```python
from build123d import *

# Parameters (mm, degrees)
F0_W     = 25.516171
F0_H     = 19.186575
F1_DEPTH = 50.8


with BuildPart() as f1:
    # F0 (on Front) → F1 (new body)
    with BuildSketch(Plane.XZ):
        with BuildLine():
            ThreePointArc((-72.431024, 58.625113), (-75.125101, 57.50919), (-76.241024, 54.815113))
            Line((-76.241024, 54.815113), (-76.241024, 3.81))
            ThreePointArc((-76.241024, 3.81), (-75.125101, 1.115923), (-72.431024, 0))
            Line((-72.431024, 0), (-65.04178, 0))
            ThreePointArc((-65.04178, 0), (-53.842533, 13.818248), (-42.643286, 0))
            Line((-42.643286, 0), (-8.830175, 0))
            ThreePointArc((-8.830175, 0), (2.476757, 13.272119), (13.783689, 0))
            Line((13.783689, 0), (49.104389, 0))
            Line((49.104389, 0), (49.104389, 27.893852))
            ThreePointArc((49.104389, 27.893852), (47.988466, 30.587929), (45.294389, 31.703852))
            Line((45.294389, 31.703852), (22.183126, 31.703852))
            Line((22.183126, 31.703852), (1.142996, 57.237982))
            ThreePointArc((1.142996, 57.237982), (-0.171807, 58.260924), (-1.797379, 58.625113))
            Line((-1.797379, 58.625113), (-72.431024, 58.625113))
        make_face()
        with Locations((-51.349548, 42.823649)):
            Rectangle(F0_W, F0_H, mode=Mode.SUBTRACT)
        Polygon((-18.218089, 33.230361), (-18.218089, 52.416936), (0, 52.416936), (14.814471, 33.230361), align=None, mode=Mode.SUBTRACT)
    extrude(amount=F1_DEPTH)


solid = f1.part
```
Input: part model. Units: mm. Frame: model coordinates. A direction names the side the tool comes from. Give positions to 0.01 mm unless a question says otherwise; leave off trailing zeros. Order: outer loops, then holes, each group sorted by start corner. A loop starts at its lowest first (then second) coordinate and runs counter-clockwise, first axis right, second up. Notation, with made-up numbers: M -5,11.5 L 28,11.5 A31 cw 28,37.5 Z; hole C 65.5,87.5 d3. An arc over 180 degrees is marked long. Return JSON: item names as keys, results as strings.
1) Mould query, pull axis Z, two halves, no side actions, for faces 1 (the face through (-52, -25, 33.23)), 2 (the face through (34, -25, 31.704)), 3 (the face through (-26, -25, 0)). Classes: released by +Z, released by -Z, zero draft, split by the parting line, or undercut.
Taken from the geometry:
{"face 1": "undercut", "face 2": "released by +Z", "face 3": "released by -Z"}
2) Section query B-B on y = -6. Output: boundary loops of the cut face in (x, z).
Taken from the geometry:
{"outline": "M -76.24,3.81 A3.81 ccw -72.43,0 L -65.04,0 A11.45 cw long -42.64,0 L -8.83,0 A11.45 cw long 13.78,0 L 49.1,0 L 49.1,27.89 A3.81 ccw 45.29,31.7 L 22.18,31.7 L 1.14,57.24 A3.81 ccw -1.8,58.63 L -72.43,58.63 A3.81 ccw -76.24,54.82 Z; hole M -64.11,33.23 L -38.59,33.23 L -38.59,52.42 L -64.11,52.42 Z; hole M -18.22,33.23 L 14.81,33.23 L 0,52.42 L -18.22,52.42 Z"}
3) Section query A-A on z = 35. Output: boundary loops of the cut face in (x, y).
Taken from the geometry:
{"outline": "M -76.24,-50.8 L -64.11,-50.8 L -64.11,0 L -76.24,0 Z; M -38.59,-50.8 L -18.22,-50.8 L -18.22,0 L -38.59,0 Z; M 13.45,-50.8 L 19.47,-50.8 L 19.47,0 L 13.45,0 Z"}
4) Contact query for flat-ended pins moving along their axis: pin 1 (13 mm diameter, centred on x = -50.5, y = -21, fed in from -Z); pin 2 (12 mm diameter, centred on x = 12.5, y = -16.5, fed in from +Z); pin 3 (9.5 mm diameter, centred on y = -15, z = 43, fed in from +X). Output: stop coordinate, or through.
Taken from the geometry:
{"pin 1": "stops at z = 8.22", "pin 2": "stops at z = 50.74", "pin 3": "stops at x = 16.79"}
5) Section query D-D on z = 6.5. Output: boundary loops of the cut face in (x, y), and give its area (3 significant figures).
Taken from the geometry:
{"outline": "M -76.24,-50.8 L -64.52,-50.8 L -64.52,0 L -76.24,0 Z; M -43.17,-50.8 L -7.98,-50.8 L -7.98,0 L -43.17,0 Z; M 12.93,-50.8 L 49.1,-50.8 L 49.1,0 L 12.93,0 Z", "area": "4,220 mm2"}
6) Section query C-C on x = 7. Output: boundary loops of the cut face in (y, z).
Taken from the geometry:
{"outline": "M -50.8,12.34 L 0,12.34 L 0,33.23 L -50.8,33.23 Z; M -50.8,43.35 L 0,43.35 L 0,50.13 L -50.8,50.13 Z"}
7) Line query: L1, parallel to Z at x = -53, y = -25.5; L2, parallel to X at y = -16.5, z = 43.5 (3 decimals); L3, parallel to X at y = -47, z = 46.5. Output: solid intervals per line, ascending. Write a range as [from, to].
Taken from the geometry:
{"L1": "z = [13.79, 33.23], [52.42, 58.63]", "L2": "x = [-76.241, -64.108], [-38.591, -18.218], [6.885, 12.463]", "L3": "x = [-76.24, -64.11], [-38.59, -18.22], [4.57, 9.99]"}
8) Access query for faces 4 (the face through (7.3, -25.04, 42.96)), 5 (the face through (-37, -25, 58.625)). Directions: +Z, -Z, +X, -X, +Y, -Y. A direction counts if a zero-diameter tool reaches every point of the face in a straight line with its end or side. Return the directions, or none.
Taken from the geometry:
{"face 4": "+Y, -Y", "face 5": "+Z, +X, -X, +Y, -Y"}
